Drawing for the job (mm, zero at the part's lowest x, y, z). Give positions to 0.01 mm unless a question says otherwise; leave off trailing zeros. Write each loop counter-clockwise with the first axis right and the second up, starting at its lowest first coordinate (ties: lowest second). Pieces come first, ordered by that corner, then holes. Notation, with made-up numbers: (-32.75, 17) - (8.25, 17) arc R24 ccw to (8.25, 53) - close; hole circle Ø4 at (26.25, 18). An arc over 180 degrees is marked (long way). Use CSV: the item, a comma, the result in double quotes.
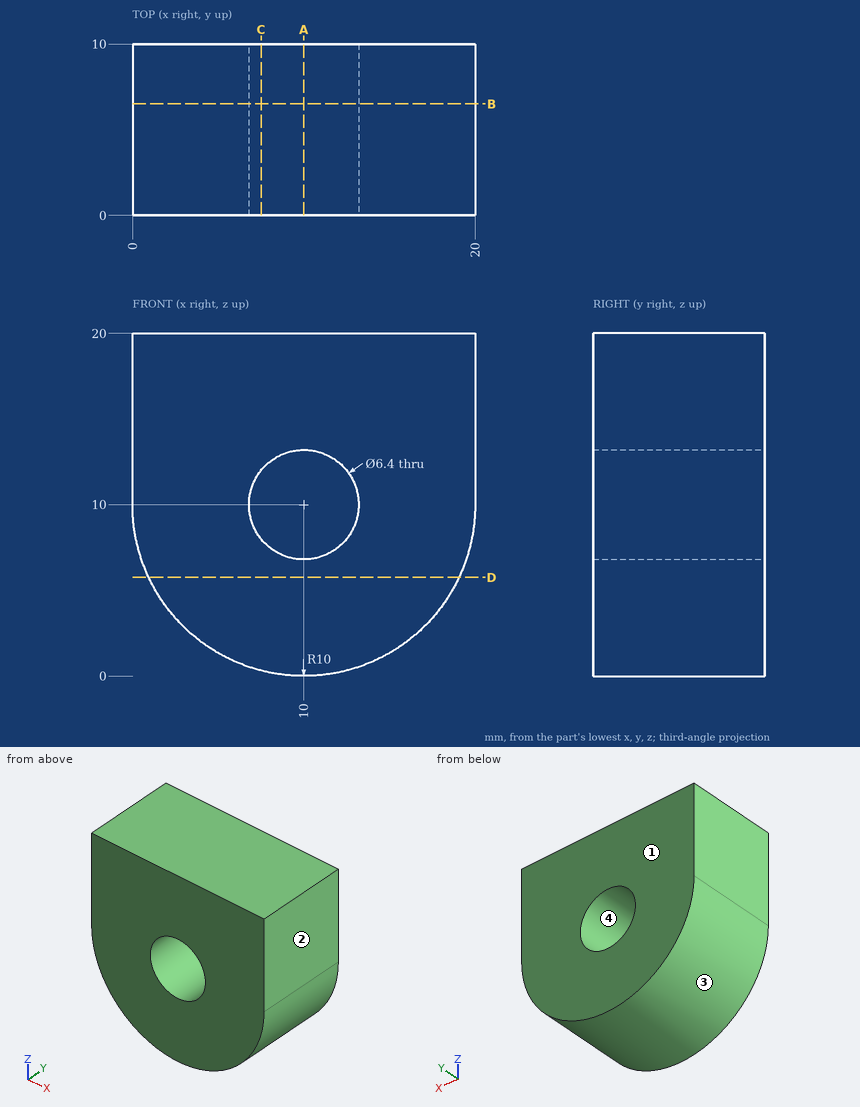
(1) Pull direction X, two halves, no side cores. Call the marked faces 1, 2, 3 and 4: released by +X, released by -X, zero draft, split by the parting line, or undercut.
Checked values:
face 1,"zero draft"
face 2,"released by +X"
face 3,"split by the parting line"
face 4,"undercut"
(2) Saw through at A-A, the plane x = 10. List the corners of the cut face in (y, z).
Checked values:
outline,"(0, 0) - (10, 0) - (10, 6.8) - (0, 6.8) - close; (0, 13.2) - (10, 13.2) - (10, 20) - (0, 20) - close"
(3) Saw through at B-B, the plane y = 6.5. List the corners of the cut face in (x, z), then the cut area to 3 significant figures.
Checked values:
outline,"(0, 10) arc R10 ccw to (20, 10) - (20, 20) - (0, 20) - close; hole circle Ø6.4 at (10, 10)"
area,"325 mm^2"
(4) Flat gauge pins, fed straight in: P1, Ø1.5, axis at y = 5, z = 4, coming from the -X side; P2, Ø2, axis at y = 3, z = 4.5, coming from the +X side; P3, Ø2, axis at x = 11, z = 9.5, coming from the -Y side. Where does each tip first touch, or does it go through?
Checked values:
P1,"stops at x = 1.49"
P2,"stops at x = 18.93"
P3,"passes through"
(5) Saw through at D-D, the plane z = 5.75. List the corners of the cut face in (x, y), then the cut area to 3 significant figures.
Checked values:
outline,"(0.95, 0) - (19.05, 0) - (19.05, 10) - (0.95, 10) - close"
area,"181 mm^2"
(6) Wall check: probe 1 along X at (y, z) = (7.25, 10); probe 2 along Z at (x, y) = (12.25, 5.5). Give the ranges that are in metal, low to high. Write a range as [from, to].
Checked values:
probe 1,"x = [0, 6.8], [13.2, 20]"
probe 2,"z = [0.26, 7.72], [12.28, 20]"
(7) Saw through at C-C, the plane x = 7.5. List the corners of the cut face in (y, z).
Checked values:
outline,"(0, 0.32) - (10, 0.32) - (10, 8) - (0, 8) - close; (0, 12) - (10, 12) - (10, 20) - (0, 20) - close"
